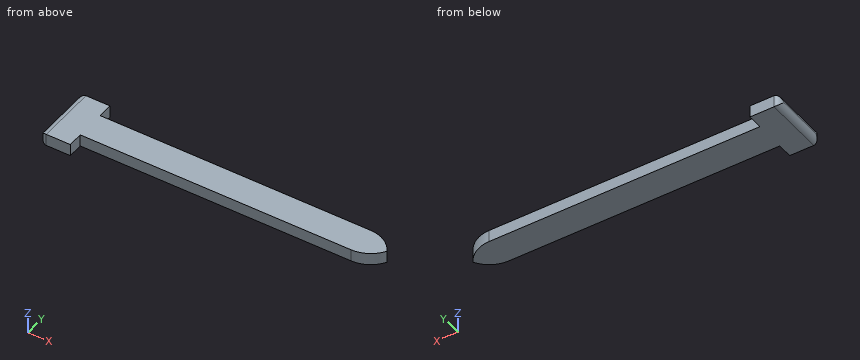
from build123d import *

# Parameters (mm, degrees)
F1_DEPTH    = 2
F2_R        = 0.99999
F3_T1_DEPTH = 27


# Not quite as in the source:
# - a fillet or chamfer that OpenCascade refuses, or shapes differently, is made with other operations: its cross-section is extruded or revolved along the edge and cut away or added
# - a fillet or chamfer is up to 0.001 mm smaller than in the source, because OpenCascade refuses the exact size


with BuildPart() as f1:
    # F0 (on Top) → F1 (new body)
    with BuildSketch(Plane.XY):
        Polygon((-25, 0), (-25, 2.5), (-25, 5), (-30, 5), (-30, -5), (-25, -5), (-25, -2.5), align=None)
        Polygon((25, -2.5), (25, 2.5), (-25, 2.5), (-25, 0), (-25, -2.5), align=None)
    extrude(amount=F1_DEPTH)

    # F2 (radius 1 in the source; OpenCascade refuses exactly that, so slightly less here)
    f2_edges = [f1.edges().sort_by_distance(p)[0] for p in [
        (-30, -5, 1),
        (-30, 0, 2),
        (-30, 5, 1),
        (-30, 0, 0),
    ]]
    fillet(f2_edges, radius=F2_R)

    # F3: fillet of radius 5 on 2 edges, made by hand

    # F3_s2 → F3_t1 (cut)
    with BuildSketch(Plane.XY.offset(-12.5)):
        with BuildLine():
            ThreePointArc((25, 2.5), (23.5355339059, -1.0355339059), (20, -2.5))
            Line((20, -2.5), (25, -2.5))
            Line((25, -2.5), (25, 2.5))
        make_face()
        with BuildLine():
            ThreePointArc((20, 2.5), (23.5355339059, 1.0355339059), (25, -2.5))
            Line((25, -2.5), (25, 2.5))
            Line((25, 2.5), (20, 2.5))
        make_face()
    extrude(amount=F3_T1_DEPTH, mode=Mode.SUBTRACT)


solid = f1.part
Model file for the job. Use its own axes, mm. Give positions to 0.01 mm unless a question says otherwise; leave off trailing zeros. Write each loop counter-clockwise with the first axis right and the second up, starting at its lowest first coordinate (ties: lowest second). Pieces come first, ordered by that corner, then holes. Notation, with made-up numbers: M 15.5,-13.5 L 38.5,-13.5 A32 ccw 38.5,15.5 Z; hole C -30,64 d3. An arc over 180 degrees is marked long. One line per item, written item: value. Start each with the question number.
Q1. Saw through at C-C, the plane z = 0.6. Write the cut outline in (x, y).
Q2. Saw through at B-B, the plane x = -14.5. Write the cut outline in (y, z).
Q3. Drop flat-ended pins along their axis: pin 1 Ø0.6 at (x, z) = (-5, 1) entering from +Y; pin 2 Ø1 at (x, z) = (8, 0.5) entering from -Y; pin 3 Ø1 at (y, z) = (3.5, 1) entering from +X. Give the stop position or say it passes through.
Q4. Probe probe 1 along Y at (x, z) = (12, 1.6); probe 2 along X at (y, z) = (4.5, 1.75); probe 3 along X at (y, z) = (-4.25, 1.35). List the from-to ranges inside material, lowest first. Write a range as [from, to].
Output values:
1. outline: M -29.92,-4.4 A1 ccw -29,-5 L -25,-5 L -25,-2.5 L 20,-2.5 A5 ccw 24.33,0 A5 ccw 20,2.5 L -25,2.5 L -25,5 L -29,5 A1 ccw -29.92,4.4 Z
2. outline: M -2.5,0 L 2.5,0 L 2.5,2 L -2.5,2 Z
3. pin 1: stops at y = 2.5
3. pin 2: stops at y = -2.5
3. pin 3: stops at x = -25
4. probe 1: y = [-2.5, 2.5]
4. probe 2: x = [-29.66, -25]
4. probe 3: x = [-29.94, -25]
